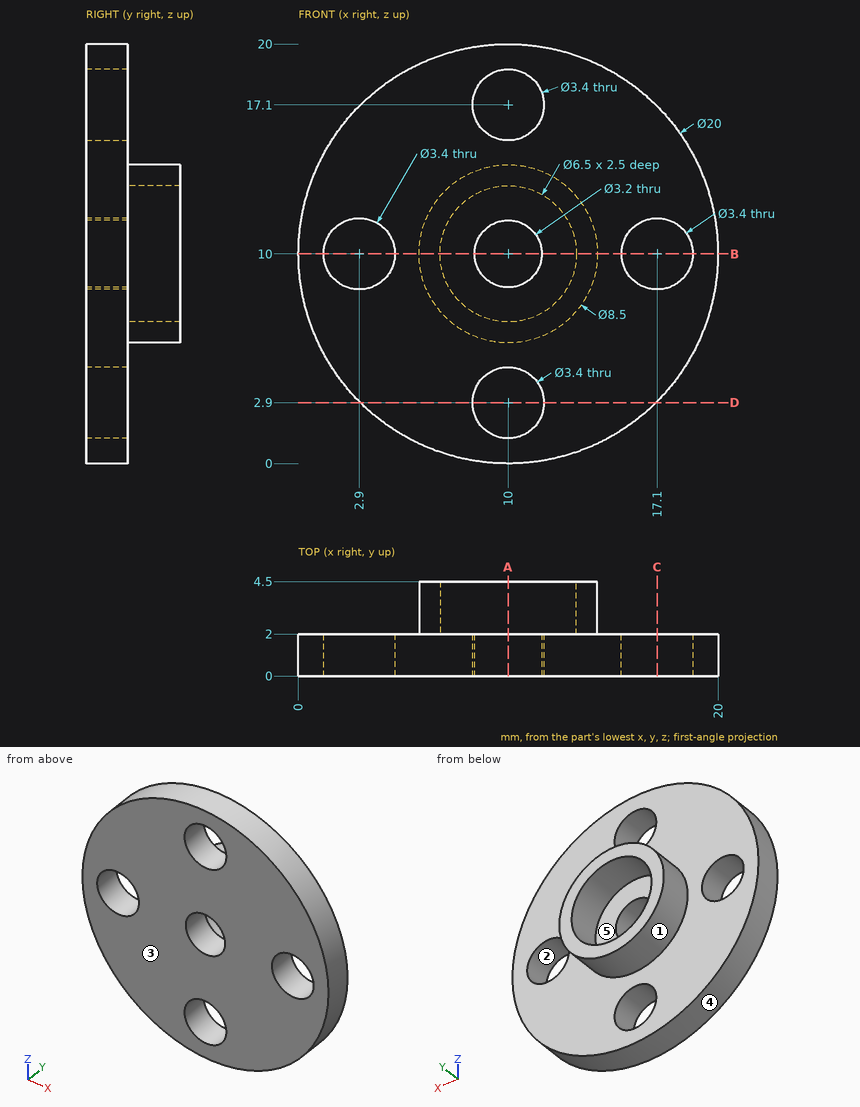
Geometry check sheet. Reference: drawing and pictorial views, mm from the part's lowest x, y, z. A direction names the side the tool comes from. Coordinates: 2 decimals unless noted, no trailing zeros. Order: outer loops, then holes, each group sorted by start corner. A loop starts at its lowest first (then second) coordinate and runs counter-clockwise, first axis right, second up. Notation, with made-up numbers: (60, 52.5) -> (93, 52.5) arc R27 cw to (93, 71.5) -> close; hole circle Ø5 at (86, 84). An arc over 180 degrees is marked (long way). Use CSV: the item, a comma, the result in double quotes. Start each with the question number.
Q1. Section check A-A, the plane x = 10. Record the cut outline in (y, z), and give its area (3 significant figures).
Q2. Draft check along X on the marked faces 3, 4 and 5. Enter one of: +X half, -X half, draft (parallel to the pull), parting line (faces both ways), or undercut.
Q3. Section check B-B, the plane z = 10. Record the cut outline in (x, y).
Q4. Section check D-D, the plane z = 2.9. Record the cut outline in (x, y), and give its area (3 significant figures).
Q5. Thickness scan on line 1 along Z through (x, y) = (10, 1.25); line 2 along Z through (x, y) = (10, 2.9). Record the ranges inside material, lowest first.
Q6. Section check C-C, the plane x = 17.1. Record the cut outline in (y, z).
Q7. Tool access check on the marked faces 1 and 2. Record the directions out of +Z, -Z, +X, -X, +Y, -Y that give a thin tool (end or side, any length) a straight path to the whole face; none if there is none.
Q8. Depth check by flat-ended pin: P1, Ø1, axis at x = 15.5, y = 0.5, coming from the +Z side; P2, Ø2, axis at y = 0.5, z = 16.5, coming from the +X side; P3, Ø2, axis at x = 11, y = 4, coming from the -Z side. Enter the tip coordinate at first touch or a pass-through.
Returned:
1,outline,"(0, 0) -> (2, 0) -> (2, 1.2) -> (0, 1.2) -> close; (0, 4.6) -> (2, 4.6) -> (2, 5.75) -> (4.5, 5.75) -> (4.5, 6.75) -> (2, 6.75) -> (2, 8.4) -> (0, 8.4) -> close; (0, 11.6) -> (2, 11.6) -> (2, 13.25) -> (4.5, 13.25) -> (4.5, 14.25) -> (2, 14.25) -> (2, 15.4) -> (0, 15.4) -> close; (0, 18.8) -> (2, 18.8) -> (2, 20) -> (0, 20) -> close"
1,area,"25.0 mm^2"
2,face 3,"draft"
2,face 4,"parting line"
2,face 5,"undercut"
3,outline,"(0, 0) -> (1.2, 0) -> (1.2, 2) -> (0, 2) -> close; (4.6, 0) -> (8.4, 0) -> (8.4, 2) -> (6.75, 2) -> (6.75, 4.5) -> (5.75, 4.5) -> (5.75, 2) -> (4.6, 2) -> close; (11.6, 0) -> (15.4, 0) -> (15.4, 2) -> (14.25, 2) -> (14.25, 4.5) -> (13.25, 4.5) -> (13.25, 2) -> (11.6, 2) -> close; (18.8, 0) -> (20, 0) -> (20, 2) -> (18.8, 2) -> close"
4,outline,"(2.96, 0) -> (8.3, 0) -> (8.3, 2) -> (2.96, 2) -> close; (11.7, 0) -> (17.04, 0) -> (17.04, 2) -> (11.7, 2) -> close"
4,area,"21.4 mm^2"
5,line 1,"z = 0 to 1.2, 4.6 to 8.4, 11.6 to 15.4, 18.8 to 20"
5,line 2,"z = 5.75 to 6.75, 13.25 to 14.25"
6,outline,"(0, 2.96) -> (2, 2.96) -> (2, 8.3) -> (0, 8.3) -> close; (0, 11.7) -> (2, 11.7) -> (2, 17.04) -> (0, 17.04) -> close"
7,face 1,"+Y"
7,face 2,"+Y, -Y"
8,P1,"stops at z = 18.66"
8,P2,"stops at x = 18.35"
8,P3,"stops at z = 5.75"
